Geometry: see drawing. Coordinates: mm, zero at the bounding-box minimum. A direction names the side the tool comes from. Round coordinates to 2 decimals unless told otherwise and drop trailing zeros. Write each loop counter-clockwise with the first axis right and the second up, starting at its lowest first coordinate (ties: lowest second). Pieces come first, ordered by that corner, then holes. Notation, with made-up numbers: M -22,-6.75 L 33,-6.75 A27 ccw 33,15.25 Z; hole C 49,71 d4. An arc over 180 degrees is marked long. Use one line per item in the form item = value. Start each with the question number.
Item 1: Ray query, probe 1 along Z at (x, y) = (5, 8); probe 2 along X at (y, z) = (8.25, 81); probe 3 along X at (y, z) = (56.6, 43). Return the intervals inside material, ascending.
Item 2: Section query B-B (x = 31.25). Return loops of the section in (y, z), and give its area (4 significant figures).
Item 3: Section query D-D (y = 33.5). Return loops of the section in (x, z).
Item 4: Section query A-A (y = 8). Return loops of the section in (x, z).
Item 5: Pin query (flat end, axial travel): pin 1 Ø7.5 at (x, z) = (4.5, 78.5) entering from +Y; pin 2 Ø3 at (x, z) = (57.5, 81) entering from -Y; pin 3 Ø4 at (x, z) = (40.5, 56.5) entering from -Y; pin 4 Ø5.5 at (y, z) = (60, 43) entering from -X. Return the tip coordinate at first contact, or that it passes through.
Item 6: Section query C-C (z = 5). Return loops of the section in (x, y), and give its area (3 significant figures).
Item 7: Pull-direction query (Z, two-part tool) for the marked faces 6 and 7; classes: pulls with the +Z half, pulls with the -Z half, needs draft (parallel to the pull), parting line crosses it, or undercut.
Item 8: Reachability of the marked faces 1, 2, 3, 4 and 5 from +Z, -Z, +X, -X, +Y, -Y: full face, straight path, thin tool, end or side. Return the list, or none.
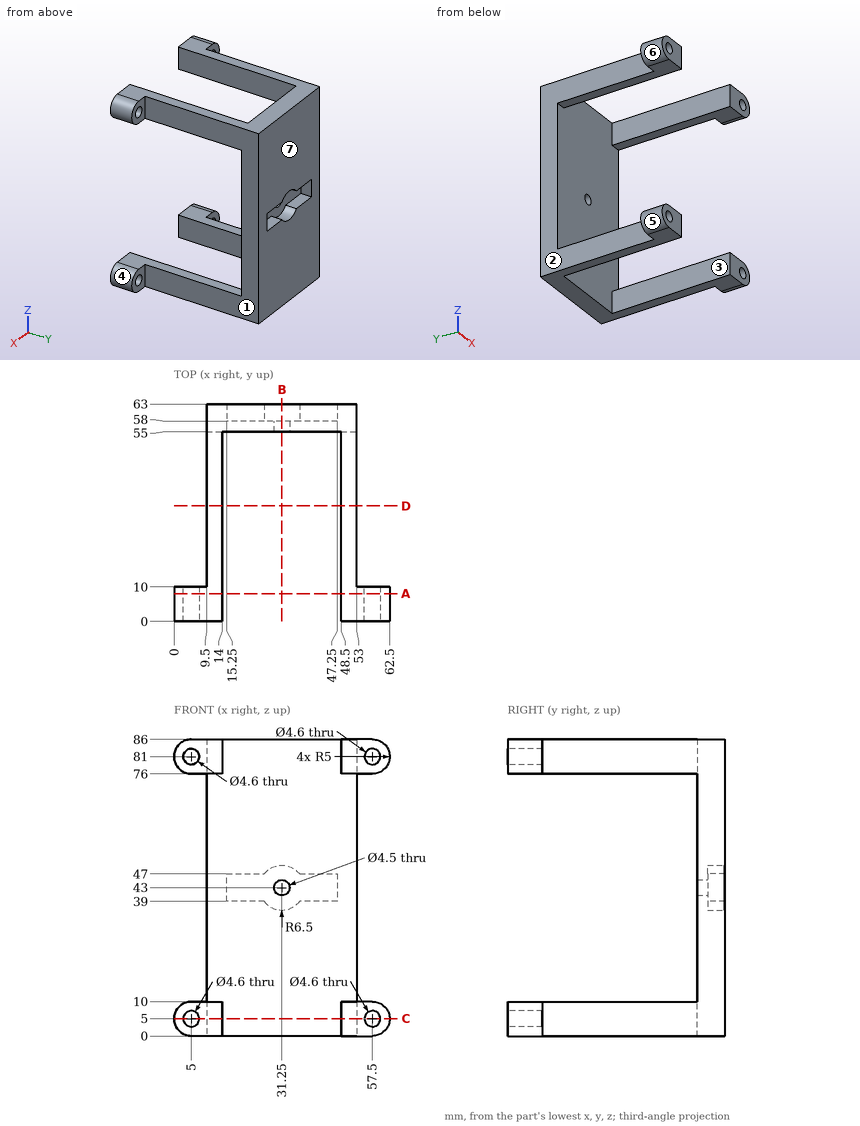
Working result:
q1.probe_1 = 0 to 2.7, 7.3 to 10, 76 to 78.7, 83.3 to 86
q1.probe_2 = 0 to 2.7, 7.3 to 14, 48.5 to 55.2, 59.8 to 62.5
q1.probe_3 = 9.5 to 29, 33.5 to 53
q2.outline = M 55,0 L 63,0 L 63,36.5 L 58,36.5 L 58,40.75 L 55,40.75 Z; M 55,45.25 L 58,45.25 L 58,49.5 L 63,49.5 L 63,86 L 55,86 Z
q2.area = 609.5 mm²
q3.outline = M 9.5,0 L 14,0 L 14,10 L 9.5,10 Z; M 9.5,76 L 14,76 L 14,86 L 9.5,86 Z; M 48.5,0 L 53,0 L 53,10 L 48.5,10 Z; M 48.5,76 L 53,76 L 53,86 L 48.5,86 Z
q4.outline = M 5,0 L 14,0 L 14,10 L 5,10 A5 ccw Z; M 5,76 L 14,76 L 14,86 L 5,86 A5 ccw Z; M 48.5,0 L 57.5,0 A5 ccw 57.5,10 L 48.5,10 Z; M 48.5,76 L 57.5,76 A5 ccw 57.5,86 L 48.5,86 Z; hole C 5,5 d4.6; hole C 5,81 d4.6; hole C 57.5,5 d4.6; hole C 57.5,81 d4.6
q5.pin_1 = 10
q5.pin_2 = through
q5.pin_3 = 55
q5.pin_4 = 9.5
q6.outline = M 0,0 L 2.7,0 L 2.7,10 L 0,10 Z; M 7.3,0 L 14,0 L 14,55 L 48.5,55 L 48.5,0 L 55.2,0 L 55.2,10 L 53,10 L 53,63 L 9.5,63 L 9.5,10 L 7.3,10 Z; M 59.8,0 L 62.5,0 L 62.5,10 L 59.8,10 Z
q6.area = 941 mm²
q7.face_6 = undercut
q7.face_7 = needs draft
q8.face_1 = +Z, -Z, +X, +Y
q8.face_2 = +Z, -Z, -X, +Y
q8.face_3 = +Z, -Z, -Y
q8.face_4 = +X, +Y, -Y
q8.face_5 = -X, +Y, -Y
